Geometry check sheet. Reference: the model listing, model coordinates, mm. Face numbers are marked on the shaded views. Coordinates: 2 decimals unless noted, no trailing zeros. Order: outer loops, then holes, each group sorted by start corner. A loop starts at its lowest first (then second) coordinate and runs counter-clockwise, first axis right, second up. Notation, with made-up numbers: (50, 69.5) - (63, 69.5) arc R26 cw to (63, 104.5) - close; hole circle Ø3 at (46.5, -25.5). An arc over 180 degrees is marked (long way). Return JSON: item names as keys, results as strings. Group by question number.
Item 1: Gauge pin test, flat ends, axial feed: pin 1 (8 mm diameter, centred on x = -5, z = 7.5, fed in from +Y); pin 2 (7 mm diameter, centred on x = -1.5, y = -1.5, fed in from +Z); pin 3 (1 mm diameter, centred on x = 2.5, z = 16.5, fed in from +Y). Record the tip position at first contact, or that the pin passes through.
Item 2: Section check B-B on z = 17.5. Enter the section's corners in (x, y).
Item 3: Scan lines: probe 1 along Y at (x, z) = (0, 11.25) (3 decimals); probe 2 along Y at (x, z) = (0, 18.25); probe 3 along X at (y, z) = (0.25, 6.25). Record each from-to range of solid material in increasing order.
Item 4: Section check C-C on z = 4.75. Enter the section's corners in (x, y) (1 decimal).
Item 5: Section check A-A on z = 11.75. Enter the section's corners in (x, y) (3 decimals).
Item 6: Draft check along Y on the marked faces 1, 2 and 3. Enter one of: pulls with the +Y half, pulls with the -Y half, needs draft (parallel to the pull), parting line crosses it, or undercut.
from build123d import *

# Parameters (mm, degrees)
F0_R     = 12.7
F1_DEPTH = 25.4
F2_T     = -1.27
F4_R     = 6.985
F5_DEPTH = 11.43
F7_R     = 1.27


# Not quite as in the source:
# - a fillet or chamfer that OpenCascade refuses, or shapes differently, is made with other operations: its cross-section is extruded or revolved along the edge and cut away or added


with BuildPart() as f1:
    # F0 (on Top) → F1 (new body)
    with BuildSketch(Plane.XY):
        Circle(F0_R)
    extrude(amount=F1_DEPTH)

    # F2
    f2_openings = [f1.faces().sort_by_distance(p)[0] for p in [
        (0, 0, 25.4),
    ]]
    offset(amount=F2_T, openings=f2_openings)

    # F4 (on offset) → F5 (join, through all)
    with BuildSketch(Plane.XY.offset(12.7)):
        Circle(F4_R)
    extrude(amount=-F5_DEPTH)

    # F6: fillet of radius 5.08 on 1 edges, made by hand

    # F6_s1 → F6_t2 (revolve)
    with BuildSketch(Plane.XZ):
        with BuildLine():
            ThreePointArc((11.43, 6.3101562476), (10.16, 2.9500520825), (6.985, 1.27))
            Line((6.985, 1.27), (11.43, 1.27))
            Line((11.43, 1.27), (11.43, 6.3101562476))
        make_face()
    revolve(axis=Axis((0, 0, 1.27), (0, 0, -1)))

    # F7
    f7_edges = [f1.edges().sort_by_distance(p)[0] for p in [
        (-6.985, 0, 1.27),
    ]]
    fillet(f7_edges, radius=F7_R)


solid = f1.part
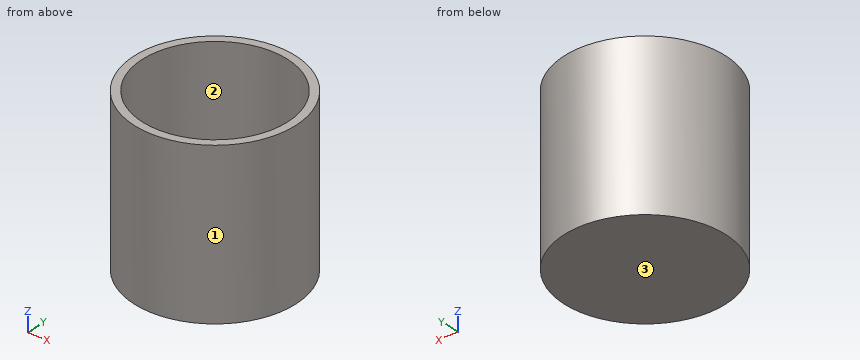
Computed:
{
 "1": {"pin 1": "stops at y = 12.66", "pin 2": "stops at z = 12.7", "pin 3": "stops at y = 12.54"},
 "2": {"outline": "circle Ø25.4 at (0, 0); hole circle Ø22.86 at (0, 0)"},
 "3": {"probe 1": "y = -12.7 to -11.43, -6.985 to 6.985, 11.43 to 12.7", "probe 2": "y = -12.7 to -11.43, 11.43 to 12.7", "probe 3": "x = -12.7 to -11.43, -6.98 to 6.98, 11.43 to 12.7"},
 "4": {"outline": "circle Ø25.4 at (0, 0); circle Ø14 at (0, 0); hole circle Ø22.4 at (0, 0)"},
 "5": {"outline": "circle Ø25.4 at (0, 0); circle Ø13.97 at (0, 0); hole circle Ø22.86 at (0, 0)"},
 "6": {"face 1": "parting line crosses it", "face 2": "undercut", "face 3": "needs draft"}
}
